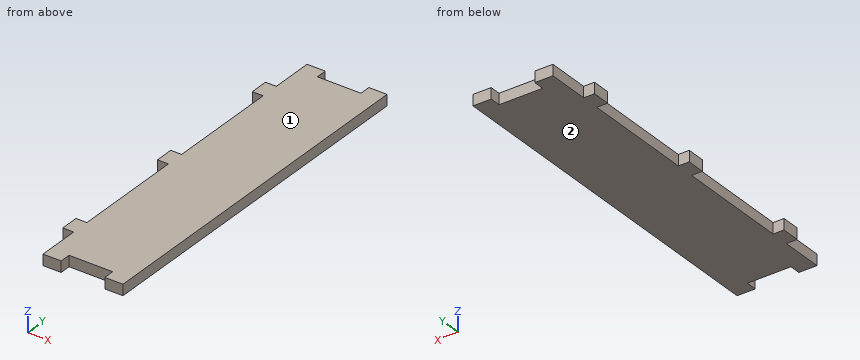
```python
from build123d import *

# Parameters (mm, degrees)
ESQUISSE1_W             = 150
ESQUISSE1_H             = 602
BOSS_EXTRU_1_DEPTH      = 18
ESQUISSE2_W             = 18
ESQUISSE2_H             = 70
ESQUISSE2_H_2           = 186
ENL_V_MAT_EXTRU_1_DEPTH = 604.224667931
ESQUISSE3_W             = 72
ESQUISSE3_H             = 18
ENL_V_MAT_EXTRU_2_DEPTH = 604.224667931


with BuildPart() as part:
    # Esquisse1 → Boss.-Extru.1 (new body)
    with BuildSketch(Plane.XY):
        with Locations((75, 283)):
            Rectangle(ESQUISSE1_W, ESQUISSE1_H)
    extrude(amount=-BOSS_EXTRU_1_DEPTH)

    # Esquisse2 → Enlèv. mat.-Extru.1 (cut, through all)
    with BuildSketch(Plane.XY):
        with Locations((9, 549)):
            Rectangle(ESQUISSE2_W, ESQUISSE2_H)
        with Locations((9, 391)):
            Rectangle(ESQUISSE2_W, ESQUISSE2_H_2)
        with Locations((9, 175)):
            Rectangle(ESQUISSE2_W, ESQUISSE2_H_2)
        with Locations((9, 17)):
            Rectangle(ESQUISSE2_W, ESQUISSE2_H)
    extrude(amount=-ENL_V_MAT_EXTRU_1_DEPTH, mode=Mode.SUBTRACT)

    # Esquisse3 → Enlèv. mat.-Extru.2 (cut, through all)
    with BuildSketch(Plane.XY):
        with Locations((84, 575)):
            Rectangle(ESQUISSE3_W, ESQUISSE3_H)
        with Locations((84, -9)):
            Rectangle(ESQUISSE3_W, ESQUISSE3_H)
    extrude(amount=-ENL_V_MAT_EXTRU_2_DEPTH, mode=Mode.SUBTRACT)


solid = part.part
```
Design review of the part built by this model. Coordinates are the model's own, in mm. Face numbers are marked on the shaded views. Coordinates: 2 decimals unless noted, no trailing zeros. Order: outer loops, then holes, each group sorted by start corner. A loop starts at its lowest first (then second) coordinate and runs counter-clockwise, first axis right, second up. Notation, with made-up numbers: M 55.5,13.5 L 85.5,13.5 A22 cw 85.5,47.5 Z; hole C 78,73 d11. An arc over 180 degrees is marked long. Answer as a JSON object with one key per item and string values. Group by question number.
1) Add section C-C, the plane x = 79.5. Write out the cut boundary in (y, z).
2) Mouldability with a two-part tool opening along Z and no side actions: class the marked faces 1 and 2 as pulls with the +Z half, pulls with the -Z half, needs draft (parallel to the pull), parting line crosses it, or undercut.
3) Wall thickness on L1, parallel to X at y = 343, z = -8.25; L2, parallel to Y at x = 58, z = -17: over which ranges is each line inside the solid? List them lowest first.
4) For pin 1 (9 mm diameter, centred on x = 83.5, z = -5, fed in from +Y); pin 2 (6 mm diameter, centred on x = 103, z = -2.5, fed in from -Y); pin 3 (5.5 mm diameter, centred on y = 556.5, z = -10.5, fed in from -X); pin 4 (4 mm diameter, centred on x = 21.5, y = 191.5, fed in from +Z), all flat-tipped, find the tip position at first contact; note any pin that passes through.
5) Add section A-A, the plane z = -11.75. Write out the cut boundary in (x, y), then the cut area to 3 significant figures.
6) Add section B-B, the plane y = 311.5. Write out the cut boundary in (x, z).
Computed values:
{
 "1": {"outline": "M 0,-18 L 566,-18 L 566,0 L 0,0 Z"},
 "2": {"face 1": "pulls with the +Z half", "face 2": "pulls with the -Z half"},
 "3": {"L1": "x = 18 to 150", "L2": "y = 0 to 566"},
 "4": {"pin 1": "stops at y = 566", "pin 2": "stops at y = 0", "pin 3": "stops at x = 18", "pin 4": "stops at z = 0"},
 "5": {"outline": "M 0,52 L 18,52 L 18,-18 L 48,-18 L 48,0 L 120,0 L 120,-18 L 150,-18 L 150,584 L 120,584 L 120,566 L 48,566 L 48,584 L 18,584 L 18,514 L 0,514 L 0,484 L 18,484 L 18,298 L 0,298 L 0,268 L 18,268 L 18,82 L 0,82 Z", "area": "78,500 mm^2"},
 "6": {"outline": "M 18,-18 L 150,-18 L 150,0 L 18,0 Z"}
}
